CAD build for the part. Positions are in the model's coordinates, mm. A direction names the side the tool comes from. Round coordinates to 2 decimals unless told otherwise and drop trailing zeros. Loops run counter-clockwise (first coordinate to the right, second up) from the corner with the lowest first, then second, coordinate; pieces in that order, holes last. Notation, with made-up numbers: M -29,16.5 L 11,16.5 A27 cw 11,44.5 Z; hole C -38.5,21.25 d11. An arc over 180 degrees is marked long. One line per item, written item: value. Start each with the question number.
from build123d import *

# Parameters (mm, degrees)
F1_DEPTH = 3
F2_DEPTH = 3


with BuildPart() as f1:
    # F0 (on Front) → F1 (new body)
    with BuildSketch(Plane.XZ):
        with BuildLine():
            Line((52.7068123221, 67.9570013285), (-77.2931876779, 67.9570013285))
            Line((-77.2931876779, 67.9570013285), (-89.2639196203, 66.7380527995))
            ThreePointArc((-89.2639196203, 66.7380527995), (-91.7316731318, 65.7829428457), (-93.3663876923, 63.7021375394))
            Line((-93.3663876923, 63.7021375394), (-99.1941262898, 49.8450988929))
            Line((-99.1941262898, 49.8450988929), (-109.0870224739, 22.5846769392))
            Line((-109.0870224739, 22.5846769392), (-120.6715287069, -11.5004989491))
            Line((-120.6715287069, -11.5004989491), (-120.6715287069, -19.3318230512))
            Line((-120.6715287069, -19.3318230512), (-118.2102517237, -24.9256293032))
            ThreePointArc((-118.2102517237, -24.9256293032), (-111.4038296451, -26.1471340573), (-106.4409637677, -21.3315948706))
            Line((-106.4409637677, -21.3315948706), (-96.8187674333, 7.0834247089))
            Line((-96.8187674333, 7.0834247089), (-93.8294616156, 20.6357413095))
            Line((-93.8294616156, 20.6357413095), (-91.3480535534, 27.9635130805))
            Line((-91.3480535534, 27.9635130805), (-87.3968608702, 30.9696110895))
            Line((-87.3968608702, 30.9696110895), (-87.0189213753, 30.9696110895))
            Line((-87.0189213753, 30.9696110895), (-87.0189213753, -23.5164099128))
            Line((-87.0189213753, -23.5164099128), (-72.0189213753, -23.5164099128))
            Line((-72.0189213753, -23.5164099128), (-72.0189213753, -9.5164099128))
            Line((-72.0189213753, -9.5164099128), (-67.7953569258, -9.5164099128))
            Line((-67.7953569258, -9.5164099128), (-67.7953569258, -23.5164099128))
            Line((-67.7953569258, -23.5164099128), (32.2046430742, -23.5164099128))
            Line((32.2046430742, -23.5164099128), (32.2046430742, -9.5164099128))
            Line((32.2046430742, -9.5164099128), (36.8044135138, -9.5164099128))
            Line((36.8044135138, -9.5164099128), (36.8044135138, -23.5164099128))
            Line((36.8044135138, -23.5164099128), (51.8044135138, -23.5164099128))
            Line((51.8044135138, -23.5164099128), (51.8044135138, 31.4835900872))
            Line((51.8044135138, 31.4835900872), (91.3881844313, 71.4835900872))
            Line((91.3881844313, 71.4835900872), (124.5390406074, 60.2576943637))
            Line((124.5390406074, 60.2576943637), (134.4878729613, 71.4835900872))
            Line((134.4878729613, 71.4835900872), (104.552151032, 98.0138096975))
            Line((104.552151032, 98.0138096975), (102.7068123221, 127.9570013285))
            Line((102.7068123221, 127.9570013285), (52.7068123221, 67.9570013285))
        make_face()
        Polygon((-85.0534210869, 30.9696110895), (-87.0189213753, 30.9696110895), (-87.0189213753, 31.4835900872), align=None, mode=Mode.SUBTRACT)
        Polygon((-78.5569989721, 29.2707944844), (-85.0534210869, 30.9696110895), (-83.5737233683, 30.9696110895), align=None, mode=Mode.SUBTRACT)
        Polygon((-87.0189213753, 31.4835900872), (-87.0189213753, 30.9696110895), (-85.0534210869, 30.9696110895), align=None)
    extrude(amount=F1_DEPTH)

    # F0 (on Front) → F2 (join)
    with BuildSketch(Plane.XZ):
        with BuildLine():
            Line((52.7068123221, 67.9570013285), (-77.2931876779, 67.9570013285))
            Line((-77.2931876779, 67.9570013285), (-89.2639196203, 66.7380527995))
            ThreePointArc((-89.2639196203, 66.7380527995), (-91.7316731318, 65.7829428457), (-93.3663876923, 63.7021375394))
            Line((-93.3663876923, 63.7021375394), (-99.1941262898, 49.8450988929))
            Line((-99.1941262898, 49.8450988929), (-109.0870224739, 22.5846769392))
            Line((-109.0870224739, 22.5846769392), (-120.6715287069, -11.5004989491))
            Line((-120.6715287069, -11.5004989491), (-120.6715287069, -19.3318230512))
            Line((-120.6715287069, -19.3318230512), (-118.2102517237, -24.9256293032))
            ThreePointArc((-118.2102517237, -24.9256293032), (-111.4038296451, -26.1471340573), (-106.4409637677, -21.3315948706))
            Line((-106.4409637677, -21.3315948706), (-96.8187674333, 7.0834247089))
            Line((-96.8187674333, 7.0834247089), (-93.8294616156, 20.6357413095))
            Line((-93.8294616156, 20.6357413095), (-91.3480535534, 27.9635130805))
            Line((-91.3480535534, 27.9635130805), (-87.3968608702, 30.9696110895))
            Line((-87.3968608702, 30.9696110895), (-87.0189213753, 30.9696110895))
            Line((-87.0189213753, 30.9696110895), (-87.0189213753, -23.5164099128))
            Line((-87.0189213753, -23.5164099128), (-72.0189213753, -23.5164099128))
            Line((-72.0189213753, -23.5164099128), (-72.0189213753, -9.5164099128))
            Line((-72.0189213753, -9.5164099128), (-67.7953569258, -9.5164099128))
            Line((-67.7953569258, -9.5164099128), (-67.7953569258, -23.5164099128))
            Line((-67.7953569258, -23.5164099128), (32.2046430742, -23.5164099128))
            Line((32.2046430742, -23.5164099128), (32.2046430742, -9.5164099128))
            Line((32.2046430742, -9.5164099128), (36.8044135138, -9.5164099128))
            Line((36.8044135138, -9.5164099128), (36.8044135138, -23.5164099128))
            Line((36.8044135138, -23.5164099128), (51.8044135138, -23.5164099128))
            Line((51.8044135138, -23.5164099128), (51.8044135138, 31.4835900872))
            Line((51.8044135138, 31.4835900872), (91.3881844313, 71.4835900872))
            Line((91.3881844313, 71.4835900872), (124.5390406074, 60.2576943637))
            Line((124.5390406074, 60.2576943637), (134.4878729613, 71.4835900872))
            Line((134.4878729613, 71.4835900872), (104.552151032, 98.0138096975))
            Line((104.552151032, 98.0138096975), (102.7068123221, 127.9570013285))
            Line((102.7068123221, 127.9570013285), (52.7068123221, 67.9570013285))
        make_face()
        Polygon((-85.0534210869, 30.9696110895), (-87.0189213753, 30.9696110895), (-87.0189213753, 31.4835900872), align=None, mode=Mode.SUBTRACT)
        Polygon((-78.5569989721, 29.2707944844), (-85.0534210869, 30.9696110895), (-83.5737233683, 30.9696110895), align=None, mode=Mode.SUBTRACT)
        Polygon((-87.0189213753, 31.4835900872), (-87.0189213753, 30.9696110895), (-85.0534210869, 30.9696110895), align=None)
    extrude(amount=F2_DEPTH)


solid = f1.part
(1) Probe L1, parallel to Z at x = 13, y = -0.7; L2, parallel to X at y = -2.25, z = -12; L3, parallel to X at y = -2.1, z = -10. List the from-to ranges inside material, lowest first.
(2) Slice it at D-D, the plane x = -20.5. List the corners of the cut face in (y, z), and give its area (3 significant figures).
(3) Which spindle directions (+Z, -Z, +X, -X, +Y, -Y) get a long thin tool onto all of the face, cutting with end or side? Do faces 1 (the flat face through (129.44, -1.48, 65.79)), 2 (the flat face through (-101.697, -1.479, -7.323)). Say none if no direction does.
(4) Slice it at C-C, the plane z = 17.5. List the corners of the cut face in (x, y).
(5) Flat gauge pins, fed straight in: P1, Ø1.5, axis at x = 41.5, y = -2, coming from the -Z side; P2, Ø1, axis at y = -2.5, z = 87, coming from the -X side; P3, Ø1, axis at x = 54, z = 2, coming from the -Y side (1 decimal); P4, Ø1.5, axis at y = -1.5, z = -1.5, coming from the -X side. Where does each tip first touch, or does it go through?
(6) Slice it at A-A, the plane z = -14. List the corners of the cut face in (x, y), and give its area (3 significant figures).
Check result:
1. L1: z = -23.52 to 67.96
1. L2: x = -120.67 to -103.28, -87.02 to -72.02, -67.8 to 32.2, 36.8 to 51.8
1. L3: x = -120.16 to -102.6, -87.02 to -72.02, -67.8 to 32.2, 36.8 to 51.8
2. outline: M -3,-23.52 L 0,-23.52 L 0,67.96 L -3,67.96 Z
2. area: 274 mm^2
3. face 1: -Z, +X, +Y, -Y
3. face 2: -Z, +Y, -Y
4. outline: M -110.82,-3 L -94.52,-3 L -94.52,0 L -110.82,0 Z; M -87.02,-3 L 51.8,-3 L 51.8,0 L -87.02,0 Z
5. P1: stops at z = -23.52
5. P2: stops at x = 68.16
5. P3: passes through
5. P4: stops at x = -117.53
6. outline: M -120.67,-3 L -103.96,-3 L -103.96,0 L -120.67,0 Z; M -87.02,-3 L -72.02,-3 L -72.02,0 L -87.02,0 Z; M -67.8,-3 L 32.2,-3 L 32.2,0 L -67.8,0 Z; M 36.8,-3 L 51.8,-3 L 51.8,0 L 36.8,0 Z
6. area: 440 mm^2
